```python
from build123d import *

# Parameters (mm, degrees)
SKETCH1_W           = 32
SKETCH1_H           = 32
SKETCH1_R           = 1.15
SKETCH1_W_2         = 13
SKETCH1_H_2         = 13
BOSS_EXTRUDE1_DEPTH = 1.6
FILLET1_R           = 2
BOSS_EXTRUDE2_DEPTH = 4
BOSS_EXTRUDE3_DEPTH = 7.75
SKETCH3_W           = 8.2
SKETCH3_H           = 3.2
BOSS_EXTRUDE4_DEPTH = 4.75


with BuildPart() as part:
    # Sketch1 → Boss-Extrude1 (new body)
    # profile 1 of 14: a face of its own
    with BuildSketch(Plane.XY):
        Rectangle(SKETCH1_W, SKETCH1_H)
        with Locations((-14, -14)):
            Circle(SKETCH1_R, mode=Mode.SUBTRACT)
        with Locations((14, -14)):
            Circle(SKETCH1_R, mode=Mode.SUBTRACT)
        with Locations((14, 14)):
            Circle(SKETCH1_R, mode=Mode.SUBTRACT)
        with Locations((-14, 14)):
            Circle(SKETCH1_R, mode=Mode.SUBTRACT)
        with BuildLine():
            ThreePointArc((-9, 2), (-11, 0), (-9, -2))
            Line((-9, -2), (9, -2))
            ThreePointArc((9, -2), (11, 0), (9, 2))
            Line((9, 2), (-9, 2))
        make_face(mode=Mode.SUBTRACT)
        Rectangle(SKETCH1_W_2, SKETCH1_H_2, mode=Mode.SUBTRACT)
    # profile 2 of 14: a face of its own
    with BuildSketch(Plane.XY):
        with BuildLine():
            Line((-6.5, 6.5), (-6.5, 2))
            Line((-6.5, 2), (-6.184658438, 2))
            ThreePointArc((-6.184658438, 2), (-3.824264641, 5.255949006), (-1.3e-08, 6.5))
            Line((-1.3e-08, 6.5), (-6.5, 6.5))
        make_face()
    # profile 3 of 14: a face of its own
    with BuildSketch(Plane.XY):
        with BuildLine():
            Line((-6.184658438, 2), (6.184658438, 2))
            ThreePointArc((6.184658438, 2), (3.82426463, 5.255949014), (-1.3e-08, 6.5))
            ThreePointArc((-1.3e-08, 6.5), (-3.824264641, 5.255949006), (-6.184658438, 2))
        make_face()
    # profile 4 of 14: a face of its own
    with BuildSketch(Plane.XY):
        with BuildLine():
            Line((6.184658438, 2), (6.5, 2))
            Line((6.5, 2), (6.5, 6.5))
            Line((6.5, 6.5), (-1.3e-08, 6.5))
            ThreePointArc((-1.3e-08, 6.5), (3.82426463, 5.255949014), (6.184658438, 2))
        make_face()
    # profile 5 of 14: a face of its own
    with BuildSketch(Plane.XY):
        with BuildLine():
            Line((6.5, 0), (6.5, -2))
            Line((6.5, -2), (9, -2))
            ThreePointArc((9, -2), (11, 0), (9, 2))
            Line((9, 2), (6.5, 2))
            Line((6.5, 2), (6.5, 0))
        make_face()
    # profile 6 of 14: a face of its own
    with BuildSketch(Plane.XY):
        with BuildLine():
            ThreePointArc((6.184658438, 2), (6.420680643, 1.01235373), (6.5, 0))
            Line((6.5, 0), (6.5, 2))
            Line((6.5, 2), (6.184658438, 2))
        make_face()
    # profile 7 of 14: a face of its own
    with BuildSketch(Plane.XY):
        with BuildLine():
            Line((6.184658438, -2), (6.5, -2))
            Line((6.5, -2), (6.5, 0))
            ThreePointArc((6.5, 0), (6.420680643, -1.01235373), (6.184658438, -2))
        make_face()
    # profile 8 of 14: a face of its own
    with BuildSketch(Plane.XY):
        with BuildLine():
            Line((1.3e-08, -6.5), (6.5, -6.5))
            Line((6.5, -6.5), (6.5, -2))
            Line((6.5, -2), (6.184658438, -2))
            ThreePointArc((6.184658438, -2), (3.824264641, -5.255949006), (1.3e-08, -6.5))
        make_face()
    # profile 9 of 14: a face of its own
    with BuildSketch(Plane.XY):
        with BuildLine():
            ThreePointArc((-6.184658438, -2), (-3.82426463, -5.255949014), (1.3e-08, -6.5))
            ThreePointArc((1.3e-08, -6.5), (3.824264641, -5.255949006), (6.184658438, -2))
            Line((6.184658438, -2), (-6.184658438, -2))
        make_face()
    # profile 10 of 14: a face of its own
    with BuildSketch(Plane.XY):
        with BuildLine():
            Line((-6.5, -6.5), (1.3e-08, -6.5))
            ThreePointArc((1.3e-08, -6.5), (-3.82426463, -5.255949014), (-6.184658438, -2))
            Line((-6.184658438, -2), (-6.5, -2))
            Line((-6.5, -2), (-6.5, -6.5))
        make_face()
    # profile 11 of 14: a face of its own
    with BuildSketch(Plane.XY):
        with BuildLine():
            Line((-9, -2), (-6.5, -2))
            Line((-6.5, -2), (-6.5, 0))
            Line((-6.5, 0), (-6.5, 2))
            Line((-6.5, 2), (-9, 2))
            ThreePointArc((-9, 2), (-11, 0), (-9, -2))
        make_face()
    # profile 12 of 14: a face of its own
    with BuildSketch(Plane.XY):
        with BuildLine():
            Line((-6.5, 2), (-6.5, 0))
            ThreePointArc((-6.5, 0), (-6.420680643, 1.01235373), (-6.184658438, 2))
            Line((-6.184658438, 2), (-6.5, 2))
        make_face()
    # profile 13 of 14: a face of its own
    with BuildSketch(Plane.XY):
        with BuildLine():
            Line((-6.5, -2), (-6.184658438, -2))
            ThreePointArc((-6.184658438, -2), (-6.420680643, -1.01235373), (-6.5, 0))
            Line((-6.5, 0), (-6.5, -2))
        make_face()
    # profile 14 of 14: a face of its own
    with BuildSketch(Plane.XY):
        with BuildLine():
            ThreePointArc((-6.5, 0), (-6.420680643, -1.01235373), (-6.184658438, -2))
            Line((-6.184658438, -2), (6.184658438, -2))
            ThreePointArc((6.184658438, -2), (6.420680643, -1.01235373), (6.5, 0))
            ThreePointArc((6.5, 0), (6.420680643, 1.01235373), (6.184658438, 2))
            Line((6.184658438, 2), (-6.184658438, 2))
            ThreePointArc((-6.184658438, 2), (-6.420680643, 1.01235373), (-6.5, 0))
        make_face()
    extrude(amount=BOSS_EXTRUDE1_DEPTH)

    # Fillet1
    fillet1_edges = [part.edges().sort_by_distance(p)[0] for p in [
        (-16, 16, 0.8),
        (16, 16, 0.8),
        (16, -16, 0.8),
        (-16, -16, 0.8),
    ]]
    fillet(fillet1_edges, radius=FILLET1_R)

    # Sketch1_3 → Boss-Extrude2 (add)
    with BuildSketch(Plane.XY):
        with BuildLine():
            Line((-6.184658438, 2), (6.184658438, 2))
            ThreePointArc((6.184658438, 2), (3.82426463, 5.255949014), (-1.3e-08, 6.5))
            ThreePointArc((-1.3e-08, 6.5), (-3.824264641, 5.255949006), (-6.184658438, 2))
        make_face()
        with BuildLine():
            Line((6.184658438, 2), (6.5, 2))
            Line((6.5, 2), (6.5, 6.5))
            Line((6.5, 6.5), (-1.3e-08, 6.5))
            ThreePointArc((-1.3e-08, 6.5), (3.82426463, 5.255949014), (6.184658438, 2))
        make_face()
        with BuildLine():
            Line((-6.5, 6.5), (-6.5, 2))
            Line((-6.5, 2), (-6.184658438, 2))
            ThreePointArc((-6.184658438, 2), (-3.824264641, 5.255949006), (-1.3e-08, 6.5))
            Line((-1.3e-08, 6.5), (-6.5, 6.5))
        make_face()
        with BuildLine():
            Line((-9, -2), (-6.5, -2))
            Line((-6.5, -2), (-6.5, 0))
            Line((-6.5, 0), (-6.5, 2))
            Line((-6.5, 2), (-9, 2))
            ThreePointArc((-9, 2), (-11, 0), (-9, -2))
        make_face()
        with BuildLine():
            ThreePointArc((-6.5, 0), (-6.420680643, -1.01235373), (-6.184658438, -2))
            Line((-6.184658438, -2), (6.184658438, -2))
            ThreePointArc((6.184658438, -2), (6.420680643, -1.01235373), (6.5, 0))
            ThreePointArc((6.5, 0), (6.420680643, 1.01235373), (6.184658438, 2))
            Line((6.184658438, 2), (-6.184658438, 2))
            ThreePointArc((-6.184658438, 2), (-6.420680643, 1.01235373), (-6.5, 0))
        make_face()
        with BuildLine():
            Line((-6.5, -6.5), (1.3e-08, -6.5))
            ThreePointArc((1.3e-08, -6.5), (-3.82426463, -5.255949014), (-6.184658438, -2))
            Line((-6.184658438, -2), (-6.5, -2))
            Line((-6.5, -2), (-6.5, -6.5))
        make_face()
        with BuildLine():
            ThreePointArc((-6.184658438, -2), (-3.82426463, -5.255949014), (1.3e-08, -6.5))
            ThreePointArc((1.3e-08, -6.5), (3.824264641, -5.255949006), (6.184658438, -2))
            Line((6.184658438, -2), (-6.184658438, -2))
        make_face()
        with BuildLine():
            Line((1.3e-08, -6.5), (6.5, -6.5))
            Line((6.5, -6.5), (6.5, -2))
            Line((6.5, -2), (6.184658438, -2))
            ThreePointArc((6.184658438, -2), (3.824264641, -5.255949006), (1.3e-08, -6.5))
        make_face()
        with BuildLine():
            ThreePointArc((6.184658438, 2), (6.420680643, 1.01235373), (6.5, 0))
            Line((6.5, 0), (6.5, 2))
            Line((6.5, 2), (6.184658438, 2))
        make_face()
        with BuildLine():
            Line((6.5, 0), (6.5, -2))
            Line((6.5, -2), (9, -2))
            ThreePointArc((9, -2), (11, 0), (9, 2))
            Line((9, 2), (6.5, 2))
            Line((6.5, 2), (6.5, 0))
        make_face()
        with BuildLine():
            Line((6.184658438, -2), (6.5, -2))
            Line((6.5, -2), (6.5, 0))
            ThreePointArc((6.5, 0), (6.420680643, -1.01235373), (6.184658438, -2))
        make_face()
        with BuildLine():
            Line((-6.5, -2), (-6.184658438, -2))
            ThreePointArc((-6.184658438, -2), (-6.420680643, -1.01235373), (-6.5, 0))
            Line((-6.5, 0), (-6.5, -2))
        make_face()
        with BuildLine():
            Line((-6.5, 2), (-6.5, 0))
            ThreePointArc((-6.5, 0), (-6.420680643, 1.01235373), (-6.184658438, 2))
            Line((-6.184658438, 2), (-6.5, 2))
        make_face()
    extrude(amount=-BOSS_EXTRUDE2_DEPTH)

    # Sketch1_4 → Boss-Extrude3 (add)
    with BuildSketch(Plane.XY):
        with BuildLine():
            Line((-6.184658438, 2), (6.184658438, 2))
            ThreePointArc((6.184658438, 2), (3.82426463, 5.255949014), (-1.3e-08, 6.5))
            ThreePointArc((-1.3e-08, 6.5), (-3.824264641, 5.255949006), (-6.184658438, 2))
        make_face()
        with BuildLine():
            ThreePointArc((-6.5, 0), (-6.420680643, -1.01235373), (-6.184658438, -2))
            Line((-6.184658438, -2), (6.184658438, -2))
            ThreePointArc((6.184658438, -2), (6.420680643, -1.01235373), (6.5, 0))
            ThreePointArc((6.5, 0), (6.420680643, 1.01235373), (6.184658438, 2))
            Line((6.184658438, 2), (-6.184658438, 2))
            ThreePointArc((-6.184658438, 2), (-6.420680643, 1.01235373), (-6.5, 0))
        make_face()
        with BuildLine():
            ThreePointArc((-6.184658438, -2), (-3.82426463, -5.255949014), (1.3e-08, -6.5))
            ThreePointArc((1.3e-08, -6.5), (3.824264641, -5.255949006), (6.184658438, -2))
            Line((6.184658438, -2), (-6.184658438, -2))
        make_face()
    extrude(amount=-BOSS_EXTRUDE3_DEPTH)

    # Sketch2 → Revolve1 (revolve)
    with BuildSketch(Plane(origin=(0, 0, 0), x_dir=(0, 0, -1), z_dir=(1, 0, 0)), mode=Mode.PRIVATE) as revolve1_sk:
        Polygon((17.95, 0), (17.95, 7), (12.95, 7), (12.95, 5.925), (7.75, 5.925), (7.75, 0), align=None)
    revolve(revolve1_sk.sketch.rotate(Axis((0, 0, 0), (0, 0, -1)), 90), axis=Axis((0, 0, 0), (0, 0, -1)))

    # Sketch3 → Boss-Extrude4 (add)
    with BuildSketch(Plane.XY.offset(1.6)):
        with Locations((6.6, -12.9)):
            Rectangle(SKETCH3_W, SKETCH3_H)
    extrude(amount=BOSS_EXTRUDE4_DEPTH)


solid = part.part
```
Work out the finished part from the listing and answer in its coordinate system (mm). A direction names the side the tool comes from. Round coordinates to 2 decimals unless told otherwise and drop trailing zeros. Write each loop counter-clockwise with the first axis right and the second up, starting at its lowest first coordinate (ties: lowest second). Pieces come first, ordered by that corner, then holes. Notation, with made-up numbers: (-25, -3) - (0, -3) arc R26 ccw to (0, 21) - close; hole circle Ø1 at (-29, 15). An arc over 180 degrees is marked (long way). Return JSON: item names as keys, results as strings. Group by question number.
Q1. Each of these flat-tipped pins is pushed along its axis until it touches: pin 1 Ø5 at (y, z) = (-5, -13) entering from +X; pin 2 Ø3 at (x, z) = (5, -4.5) entering from +Y; pin 3 Ø3.5 at (y, z) = (-13.5, 3.5) entering from +X. Where does it stop, or does it pass through?
Q2. The part is cut by section A-A on z = 0.5. Write down the section's boundary in (x, y), then the cut area to 3 significant figures.
Q3. For faces 1 (the cylindrical face through (5.65, -1.78, -10.31)), 2 (the flat face through (10.7, -13, 4)), 3 (the flat face through (0, 6.5, -2)), 4 (the flat face through (0, -6.5, -2)), determine the directions among +Z, -Z, +X, -X, +Y, -Y from which every point of the face is accessible in a straight line to the end or side of a thin tool.
Q4. Find the intervals of material crossed by L1, parallel to Y at x = 14, z = 1.1; L2, parallel to Z at x = 8, y = 6.5; L3, parallel to Z at x = -3, y = -0.5, in increasing order.
Q5. The part is cut by section D-D on x = 13.5. Write down the section's boundary in (y, z).
Q6. The part is cut by section C-C on y = -12. Write down the section's boundary in (x, z), then the cut area to 4 significant figures.
Q7. The mould has two halves that part along Z. Classify faces 5 (the flat face through (7, -13, 6.35)), 6 (the flat face through (0, -16, 1)), 7 (the flat face through (-6, -2, -12.95)): released by +Z, released by -Z, zero draft, split by the parting line, or undercut.
Q8. The part is cut by section B-B on x = -8. Write down the section's boundary in (y, z).
Solved:
{
 "1": {"pin 1": "x = 6.54", "pin 2": "y = 6.5", "pin 3": "x = 10.7"},
 "2": {"outline": "(-16, -14) arc R2 ccw to (-14, -16) - (14, -16) arc R2 ccw to (16, -14) - (16, 14) arc R2 ccw to (14, 16) - (-14, 16) arc R2 ccw to (-16, 14) - close; hole circle Ø2.3 at (-14, -14); hole circle Ø2.3 at (-14, 14); hole circle Ø2.3 at (14, -14); hole circle Ø2.3 at (14, 14)", "area": "1,000 mm²"},
 "3": {"face 1": "none", "face 2": "+Z, +X, +Y, -Y", "face 3": "+X, -X, +Y", "face 4": "+X, -X, -Y"},
 "4": {"L1": "-16 to -15.15, -12.85 to 12.85, 15.15 to 16", "L2": "0 to 1.6", "L3": "-17.95 to 1.6"},
 "5": {"outline": "(-16, 0) - (-15.04, 0) - (-15.04, 1.6) - (-16, 1.6) - close; (-12.96, 0) - (12.96, 0) - (12.96, 1.6) - (-12.96, 1.6) - close; (15.04, 0) - (16, 0) - (16, 1.6) - (15.04, 1.6) - close"},
 "6": {"outline": "(-16, 0) - (16, 0) - (16, 1.6) - (10.7, 1.6) - (10.7, 6.35) - (2.5, 6.35) - (2.5, 1.6) - (-16, 1.6) - close", "area": "90.15 mm²"},
 "7": {"face 5": "released by +Z", "face 6": "zero draft", "face 7": "undercut"},
 "8": {"outline": "(-16, 0) - (-2, 0) - (-2, -4) - (2, -4) - (2, 0) - (16, 0) - (16, 1.6) - (-16, 1.6) - close"}
}
